```python
from build123d import *

# Parameters (mm, degrees)
F1_DEPTH = 16
F3_START = -1.5
F2_W     = 13
F2_H     = 49.3902075756
F2_W_2   = 53.9163745879
F2_H_2   = 13
F3_DEPTH = 13


with BuildPart() as f1:
    # F0 (on Front) → F1 (new body)
    with BuildSketch(Plane.XZ):
        Polygon((0, 60), (0, 0), (60, 0), align=None)
    extrude(amount=F1_DEPTH)

    # F2 (on face) → F3 (cut)
    with BuildSketch(Plane(origin=(0, 0, 0), x_dir=(-1, 0, 0), z_dir=(0, 1, 0)).offset(F3_START)):
        with Locations((-8.3, 44.6951037878)):
            Rectangle(F2_W, F2_H)
        with Locations((-46.958187294, 8.3)):
            Rectangle(F2_W_2, F2_H_2)
    extrude(amount=-F3_DEPTH, mode=Mode.SUBTRACT)


solid = f1.part
```
The listing builds one solid part. Answer for the finished solid, in the listing's coordinates (mm). A direction names the side the tool comes from. Coordinates: 2 decimals unless noted, no trailing zeros. Loops run counter-clockwise (first coordinate to the right, second up) from the corner with the lowest first, then second, coordinate; pieces in that order, holes last. Notation, with made-up numbers: M 88,-9.5 L 104,-9.5 A22 ccw 104,16.5 Z; hole C 68.5,-5 d5. An arc over 180 degrees is marked long. Answer as a JSON object with one key per item and string values. Group by question number.
Item 1: Section B-B (x = 41) is taken. Write down the section's boundary in (y, z), and give its area (3 significant figures).
Item 2: Section A-A (z = 42.5) is taken. Write down the section's boundary in (x, y).
Item 3: Each of these flat-tipped pins is pushed along its axis until it touches: P1, Ø4, axis at x = 30, y = -9, coming from the +Z side; P2, Ø8, axis at x = 10.5, y = -10, coming from the +Z side; P3, Ø6.5, axis at y = -11, z = 37, coming from the +X side. Where does it stop, or does it pass through?
Item 4: Section D-D (y = -11.5) is taken. Write down the section's boundary in (x, z).
Item 5: Determine the mould class of faces 4 (the face through (30, -8, 30)), 5 (the face through (20, -8, 8)), 6 (the face through (1.8, -8, 39)) for opening direction Z: +Z half, -Z half, draft (parallel to the pull), parting line (faces both ways), or undercut.
Item 6: Which of the six approach directions +Z, -Z, +X, -X, +Y, -Y give full straight-line access (tool end or side, diameter ignored) to faces 1 (the face through (16, -16, 17)), 2 (the face through (33, -8, 14.8)), 3 (the face through (8, -8, 20))?
Item 7: Section C-C (x = 6) is taken. Write down the section's boundary in (y, z), and give its area (3 significant figures).
Item 8: Consider L1, parallel to Z at x = 40, y = -3.5; L2, parallel to Y at x = 5, z = 25; L3, parallel to Z at x = 47, y = -11.25. Determine where each line is inside the solid, lowest interval first.
Solved:
{
 "1": {"outline": "M -16,0 L 0,0 L 0,19 L -16,19 Z; hole M -14.5,1.8 L -1.5,1.8 L -1.5,14.8 L -14.5,14.8 Z", "area": "135 mm2"},
 "2": {"outline": "M 0,-16 L 17.5,-16 L 17.5,0 L 0,0 Z; hole M 1.8,-14.5 L 14.8,-14.5 L 14.8,-1.5 L 1.8,-1.5 Z"},
 "3": {"P1": "stops at z = 32", "P2": "stops at z = 20", "P3": "stops at x = 26.25"},
 "4": {"outline": "M 0,0 L 60,0 L 58.2,1.8 L 20,1.8 L 20,14.8 L 45.2,14.8 L 14.8,45.2 L 14.8,20 L 1.8,20 L 1.8,58.2 L 0,60 Z"},
 "5": {"face 4": "+Z half", "face 5": "undercut", "face 6": "draft"},
 "6": {"face 1": "+Z, -Z, +X, -X, -Y", "face 2": "+X", "face 3": "+Z"},
 "7": {"outline": "M -16,0 L 0,0 L 0,54 L -1.5,54 L -1.5,20 L -14.5,20 L -14.5,54 L -16,54 Z", "area": "422 mm2"},
 "8": {"L1": "z = 0 to 1.8, 14.8 to 20", "L2": "y = -16 to -14.5, -1.5 to 0", "L3": "z = 0 to 1.8"}
}
